```python
from build123d import *

# Parameters (mm, degrees)
F1_DEPTH = 209.55
F2_W     = 20.6375
F2_H     = 20.6375
F2_W_2   = 69.85
F2_H_2   = 55.5625
F3_DEPTH = 0.4064


# Not quite as in the source:
# - the dataset's text gives a spline's control points without its knots; the knots are read off the source's solid


with BuildPart() as f1:
    # F0 (on Right) → F1 (new body, symmetric)
    with BuildSketch(Plane.YZ):
        Polygon((-139.7, 0), (0, 0), (0, 50.8), (-139.2936, 50.8), (-139.2936, 51.054), (-40.6298144724, 149.7177855276), (-40.9171826682, 150.0051537235), (-139.7, 51.2223363917), align=None)
    extrude(amount=F1_DEPTH, both=True)

    # F2 (on face) → F3 (cut, through all)
    with BuildSketch(Plane(origin=(0, -95.4611681959, 95.4611681959), x_dir=(1, 0, 0), z_dir=(0, -0.7071067812, 0.7071067812))):
        with Locations((52.3081513166, -13.6913588034)):
            Rectangle(F2_W, F2_H)
        with Locations((139.6206513166, 40.2836411966)):
            Rectangle(F2_W_2, F2_H_2)
        with Locations((22.1456513166, 40.2836411966)):
            Rectangle(F2_W_2, F2_H_2)
        with BuildLine():
            add(Edge.make_bspline(
                [(-69.2965076834, -25.7584924034), (-66.1370016834, -28.9176682034), (-61.6969800834, -30.7569838034), (-57.2293486834, -30.7569838034), (-52.7614378834, -30.7569838034), (-48.3210606834, -28.9176682034), (-45.1618848834, -25.7584924034), (-42.0027344834, -22.5993420034), (-40.1637236834, -18.1593204034), (-40.1637236834, -13.6913588034), (-40.1637236834, -9.2234226034), (-42.0027344834, -4.7833502034), (-45.1618848834, -1.6242252034), (-48.3210606834, 1.5349251966), (-52.7614378834, 3.3742661966), (-57.2293486834, 3.3742661966)],
                knots=[3, 3, 3, 3, 4, 4, 4, 5, 5, 5, 6, 6, 6, 7, 7, 7, 8, 8, 8, 8], degree=3))
            add(Edge.make_bspline(
                [(-57.2293486834, 3.3742661966), (-61.6969800834, 3.3742661966), (-66.1370016834, 1.5349251966), (-69.2965076834, -1.6242252034)],
                knots=[0, 0, 0, 0, 1, 1, 1, 1], degree=3))
            add(Edge.make_bspline(
                [(-69.2965076834, -1.6242252034), (-72.4556326834, -4.7833502034), (-74.2949736834, -9.2234226034), (-74.2949736834, -13.6913588034), (-74.2949736834, -18.1593204034), (-72.4556326834, -22.5993420034), (-69.2965076834, -25.7584924034)],
                knots=[1, 1, 1, 1, 2, 2, 2, 3, 3, 3, 3], degree=3))
        make_face()
        with BuildLine():
            add(Edge.make_bspline(
                [(82.0141371166, 11.2521523966), (80.4710871166, 12.7948975966), (78.3027399166, 13.6930161966), (76.1206513166, 13.6930161966)],
                knots=[7, 7, 7, 7, 8, 8, 8, 8], degree=3))
            add(Edge.make_bspline(
                [(76.1206513166, 13.6930161966), (73.9388421166, 13.6930161966), (71.7701901166, 12.7948975966), (70.2274449166, 11.2521523966)],
                knots=[0, 0, 0, 0, 1, 1, 1, 1], degree=3))
            add(Edge.make_bspline(
                [(70.2274449166, 11.2521523966), (68.6847505166, 9.7091023966), (67.7862763166, 7.5404503966), (67.7862763166, 5.3586411966), (67.7862763166, 3.1768573966), (68.6847505166, 1.0081545966), (70.2274449166, -0.5345398034)],
                knots=[1, 1, 1, 1, 2, 2, 2, 3, 3, 3, 3], degree=3))
            add(Edge.make_bspline(
                [(70.2274449166, -0.5345398034), (71.7701901166, -2.0775898034), (73.9388421166, -2.9757338034), (76.1206513166, -2.9757338034), (78.3027399166, -2.9757338034), (80.4710871166, -2.0775898034), (82.0141371166, -0.5345398034)],
                knots=[3, 3, 3, 3, 4, 4, 4, 5, 5, 5, 5], degree=3))
            add(Edge.make_bspline(
                [(82.0141371166, -0.5345398034), (83.5572379166, 1.0081545966), (84.4550263166, 3.1768573966), (84.4550263166, 5.3586411966), (84.4550263166, 7.5404503966), (83.5572379166, 9.7091023966), (82.0141371166, 11.2521523966)],
                knots=[5, 5, 5, 5, 6, 6, 6, 7, 7, 7, 7], degree=3))
        make_face()
        with BuildLine():
            add(Edge.make_bspline(
                [(-68.0362866834, 54.8767285966), (-71.8565482834, 58.6969901966), (-77.2264130834, 60.9211411966), (-82.6293486834, 60.9211411966)],
                knots=[7, 7, 7, 7, 8, 8, 8, 8], degree=3))
            add(Edge.make_bspline(
                [(-82.6293486834, 60.9211411966), (-88.0319794834, 60.9211411966), (-93.4014886834, 58.6969901966), (-97.2220804834, 54.8767285966)],
                knots=[0, 0, 0, 0, 1, 1, 1, 1], degree=3))
            add(Edge.make_bspline(
                [(-97.2220804834, 54.8767285966), (-101.0426976834, 51.0561113966), (-103.2668486834, 45.6865767966), (-103.2668486834, 40.2836411966), (-103.2668486834, 34.8807055966), (-101.0426976834, 29.5111455966), (-97.2220804834, 25.6905791966)],
                knots=[1, 1, 1, 1, 2, 2, 2, 3, 3, 3, 3], degree=3))
            add(Edge.make_bspline(
                [(-97.2220804834, 25.6905791966), (-93.4014886834, 21.8703175966), (-88.0319794834, 19.6461411966), (-82.6293486834, 19.6461411966), (-77.2264130834, 19.6461411966), (-71.8565482834, 21.8703175966), (-68.0362866834, 25.6905791966)],
                knots=[3, 3, 3, 3, 4, 4, 4, 5, 5, 5, 5], degree=3))
            add(Edge.make_bspline(
                [(-68.0362866834, 25.6905791966), (-64.2160250834, 29.5111455966), (-61.9918486834, 34.8807055966), (-61.9918486834, 40.2836411966), (-61.9918486834, 45.6865767966), (-64.2160250834, 51.0561113966), (-68.0362866834, 54.8767285966)],
                knots=[5, 5, 5, 5, 6, 6, 6, 7, 7, 7, 7], degree=3))
        make_face()
        with BuildLine():
            add(Edge.make_bspline(
                [(-160.1112866834, 54.8767285966), (-163.9315482834, 58.6969901966), (-169.3014130834, 60.9211411966), (-174.7043486834, 60.9211411966)],
                knots=[7, 7, 7, 7, 8, 8, 8, 8], degree=3))
            add(Edge.make_bspline(
                [(-174.7043486834, 60.9211411966), (-180.1069794834, 60.9211411966), (-185.4764886834, 58.6969901966), (-189.2970804834, 54.8767285966)],
                knots=[0, 0, 0, 0, 1, 1, 1, 1], degree=3))
            add(Edge.make_bspline(
                [(-189.2970804834, 54.8767285966), (-193.1176976834, 51.0561113966), (-195.3418486834, 45.6865767966), (-195.3418486834, 40.2836411966), (-195.3418486834, 34.8807055966), (-193.1176976834, 29.5111455966), (-189.2970804834, 25.6905791966)],
                knots=[1, 1, 1, 1, 2, 2, 2, 3, 3, 3, 3], degree=3))
            add(Edge.make_bspline(
                [(-189.2970804834, 25.6905791966), (-185.4764886834, 21.8703175966), (-180.1069794834, 19.6461411966), (-174.7043486834, 19.6461411966), (-169.3014130834, 19.6461411966), (-163.9315482834, 21.8703175966), (-160.1112866834, 25.6905791966)],
                knots=[3, 3, 3, 3, 4, 4, 4, 5, 5, 5, 5], degree=3))
            add(Edge.make_bspline(
                [(-160.1112866834, 25.6905791966), (-156.2910250834, 29.5111455966), (-154.0668486834, 34.8807055966), (-154.0668486834, 40.2836411966), (-154.0668486834, 45.6865767966), (-156.2910250834, 51.0561113966), (-160.1112866834, 54.8767285966)],
                knots=[5, 5, 5, 5, 6, 6, 6, 7, 7, 7, 7], degree=3))
        make_face()
        with BuildLine():
            add(Edge.make_bspline(
                [(-133.1194686834, -3.0270418034), (-135.9113858834, -0.2354802034), (-139.8353556834, 1.3898911966), (-143.7837856834, 1.3898911966)],
                knots=[7, 7, 7, 7, 8, 8, 8, 8], degree=3))
            add(Edge.make_bspline(
                [(-143.7837856834, 1.3898911966), (-147.7318600834, 1.3898911966), (-151.6558044834, -0.2354802034), (-154.4477216834, -3.0270418034)],
                knots=[0, 0, 0, 0, 1, 1, 1, 1], degree=3))
            add(Edge.make_bspline(
                [(-154.4477216834, -3.0270418034), (-157.2396388834, -5.8189844034), (-158.8650356834, -9.7429288034), (-158.8650356834, -13.6913588034), (-158.8650356834, -17.6397888034), (-157.2396388834, -21.5637332034), (-154.4477216834, -24.3552948034)],
                knots=[1, 1, 1, 1, 2, 2, 2, 3, 3, 3, 3], degree=3))
            add(Edge.make_bspline(
                [(-154.4477216834, -24.3552948034), (-151.6558044834, -27.1472120034), (-147.7318600834, -28.7726088034), (-143.7837856834, -28.7726088034), (-139.8353556834, -28.7726088034), (-135.9113858834, -27.1472120034), (-133.1194686834, -24.3552948034), (-130.3279070834, -21.5637332034), (-128.7025356834, -17.6397888034), (-128.7025356834, -13.6913588034), (-128.7025356834, -9.7429288034), (-130.3279070834, -5.8189844034), (-133.1194686834, -3.0270418034)],
                knots=[3, 3, 3, 3, 4, 4, 4, 5, 5, 5, 6, 6, 6, 7, 7, 7, 7], degree=3))
        make_face()
        with BuildLine():
            add(Edge.make_bspline(
                [(176.2819699166, -8.7803704034), (174.9962473166, -7.4946732034), (173.1889611166, -6.7460336034), (171.3706513166, -6.7460336034)],
                knots=[7, 7, 7, 7, 8, 8, 8, 8], degree=3))
            add(Edge.make_bspline(
                [(171.3706513166, -6.7460336034), (169.5523161166, -6.7460336034), (167.7453601166, -7.4946732034), (166.4596629166, -8.7803704034)],
                knots=[0, 0, 0, 0, 1, 1, 1, 1], degree=3))
            add(Edge.make_bspline(
                [(166.4596629166, -8.7803704034), (165.1739657166, -10.0660930034), (164.4253261166, -11.8730236034), (164.4253261166, -13.6913588034), (164.4253261166, -15.5096686034), (165.1739657166, -17.3166246034), (166.4596629166, -18.6023218034)],
                knots=[1, 1, 1, 1, 2, 2, 2, 3, 3, 3, 3], degree=3))
            add(Edge.make_bspline(
                [(166.4596629166, -18.6023218034), (167.7453601166, -19.8880444034), (169.5523161166, -20.6366586034), (171.3706513166, -20.6366586034), (173.1889611166, -20.6366586034), (174.9962473166, -19.8880444034), (176.2819699166, -18.6023218034), (177.5676671166, -17.3166246034), (178.3159511166, -15.5096686034), (178.3159511166, -13.6913588034), (178.3159511166, -11.8730236034), (177.5676671166, -10.0660930034), (176.2819699166, -8.7803704034)],
                knots=[3, 3, 3, 3, 4, 4, 4, 5, 5, 5, 6, 6, 6, 7, 7, 7, 7], degree=3))
        make_face()
        with BuildLine():
            add(Edge.make_bspline(
                [(198.3663809166, 10.1293961966), (197.1175645166, 11.3782633966), (195.3622721166, 12.1055161966), (193.5956513166, 12.1055161966)],
                knots=[7, 7, 7, 7, 8, 8, 8, 8], degree=3))
            add(Edge.make_bspline(
                [(193.5956513166, 12.1055161966), (191.8293607166, 12.1055161966), (190.0740683166, 11.3782633966), (188.8248709166, 10.1293961966)],
                knots=[0, 0, 0, 0, 1, 1, 1, 1], degree=3))
            add(Edge.make_bspline(
                [(188.8248709166, 10.1293961966), (187.5760037166, 8.8805797966), (186.8487763166, 7.1249317966), (186.8487763166, 5.3586411966), (186.8487763166, 3.5923251966), (187.5760037166, 1.8367279966), (188.8248709166, 0.5878607966)],
                knots=[1, 1, 1, 1, 2, 2, 2, 3, 3, 3, 3], degree=3))
            add(Edge.make_bspline(
                [(188.8248709166, 0.5878607966), (190.0740683166, -0.6609810034), (191.8293607166, -1.3882338034), (193.5956513166, -1.3882338034), (195.3622721166, -1.3882338034), (197.1175645166, -0.6609810034), (198.3663809166, 0.5878607966)],
                knots=[3, 3, 3, 3, 4, 4, 4, 5, 5, 5, 5], degree=3))
            add(Edge.make_bspline(
                [(198.3663809166, 0.5878607966), (199.6155783166, 1.8367279966), (200.3425263166, 3.5923251966), (200.3425263166, 5.3586411966), (200.3425263166, 7.1249317966), (199.6155783166, 8.8805797966), (198.3663809166, 10.1293961966)],
                knots=[5, 5, 5, 5, 6, 6, 6, 7, 7, 7, 7], degree=3))
        make_face()
    extrude(amount=-F3_DEPTH, mode=Mode.SUBTRACT)


solid = f1.part
```
Check sheet for the modelled part. Datum: model origin and axes. Units: mm. A direction names the side the tool comes from. Round coordinates to 2 decimals unless told otherwise and drop trailing zeros. Loops run counter-clockwise (first coordinate to the right, second up) from the corner with the lowest first, then second, coordinate; pieces in that order, holes last. Notation, with made-up numbers: (62, -28.5) - (90, -28.5) arc R10 ccw to (90, -12.5) - close; hole circle Ø9 at (-23, 4). An arc over 180 degrees is marked (long way). Answer as a JSON object with one key per item and string values. Group by question number.
Q1. Sectioned sample at D-D, the plane y = -17. Enter the section's corners in (x, z).
Q2. Sectioned sample at C-C, the plane x = 95. Enter the section's corners in (y, z).
Q3. Gauge pin test, flat ends, axial feed: P1, Ø4, axis at x = 93, y = -78.5, coming from the +Z side; P2, Ø6, axis at x = 33, z = 77, coming from the +Y side; P3, Ø1, axis at x = -51.5, z = 102, coming from the +Y side. Record the tip position at first contact, or that the pin passes through.
Q4. Set-up check for faces 4 (the face through (-12.779, -67.1, 123.5)), 5 (the face through (3, 0, 25)), 6 (the face through (2.93, -90.65, 99.7)): record each of +Z, -Z, +X, -X, +Y, -Y from which the full face is reachable in a straight line by a thin tool's end or side.
Q5. Mould release check, pull along X, two halves, no side actions. Record for faces 1 (the face through (209.55, -70, 31)), 2 (the face through (174.546, -67.1, 123.5)), 3 (the face through (3, -139.7, 26)): released by +X, released by -X, zero draft, split by the parting line, or undercut.
Q6. Scan lines: line 1 along Z through (x, y) = (181.5, -7); line 2 along Y through (x, z) = (-131, 93); line 3 along Z through (x, y) = (82.5, -47). Record each from-to range of solid material in increasing order. Write a range as [from, to].
Q7. Sectioned sample at A-A, the plane x = 32. Enter the section's corners in (y, z).
Q8. Sectioned sample at B-B, the plane y = -124.5. Enter the section's corners in (x, z), plus the area to 3 significant figures.
Solution:
{
 "1": {"outline": "(-209.55, 0) - (209.55, 0) - (209.55, 50.8) - (-209.55, 50.8) - close"},
 "2": {"outline": "(-139.7, 0) - (0, 0) - (0, 50.8) - (-139.29, 50.8) - (-139.29, 51.05) - (-40.63, 149.72) - (-40.92, 150.01) - (-139.7, 51.22) - close"},
 "3": {"P1": "stops at z = 114.42", "P2": "stops at y = -110.35", "P3": "stops at y = -87.85"},
 "4": {"face 4": "+Z, +Y, -Y", "face 5": "+Z, -Z, +X, -X, +Y", "face 6": "+X, -X, +Y"},
 "5": {"face 1": "released by +X", "face 2": "undercut", "face 3": "zero draft"},
 "6": {"line 1": "z = [0, 50.8]", "line 2": "y = [-97.92, -97.35]", "line 3": "z = [0, 50.8], [143.35, 143.92]"},
 "7": {"outline": "(-139.7, 0) - (0, 0) - (0, 50.8) - (-139.29, 50.8) - (-139.29, 51.05) - (-86.33, 104.01) - (-86.62, 104.3) - (-139.7, 51.22) - close; (-47.33, 143.59) - (-47.04, 143.3) - (-40.63, 149.72) - (-40.92, 150.01) - close"},
 "8": {"outline": "(-209.55, 0) - (209.55, 0) - (209.55, 50.8) - (-209.55, 50.8) - close; (-209.55, 65.85) - (209.55, 65.85) - (209.55, 66.42) - (-209.55, 66.42) - close", "area": "21,500 mm²"}
}
